Verification items for the finished model (mm, model axes). Coordinates: 2 decimals unless noted, no trailing zeros. Order: outer loops, then holes, each group sorted by start corner. A loop starts at its lowest first (then second) coordinate and runs counter-clockwise, first axis right, second up. Notation, with made-up numbers: M -3.75,82 L 32.25,82 A24 cw 32.25,119 Z; hole C 75,5.5 d4. An arc over 180 degrees is marked long. Return JSON: item names as keys, results as strings.
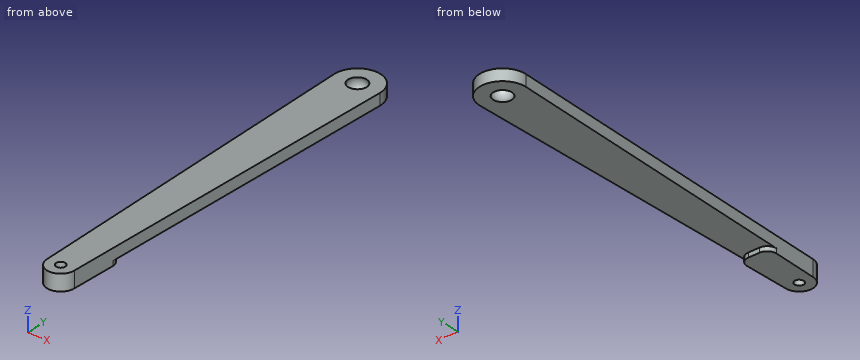
Autodesk Inventor part; units mm, degrees
ref_plane "YZ Plane" through (0, 0, 0) normal (1, 0, 0) x (0, 1, 0)
ref_plane "XZ Plane" through (0, 0, 0) normal (0, 1, 0) x (-1, 0, 0)
ref_plane "XY Plane" through (0, 0, 0) normal (0, 0, 1) x (1, 0, 0)
sketch "Sketch1" plane through (0, 0, 0) normal (0, 0, 1) x (1, 0, 0)
  circle A0 centre (0, 0) radius 0.5
  spline S0 degree 3 poles (0.2195, 78.8895) (0.2199, 78.9523) (0.2329, 79.0192) (0.2847, 79.142) (0.3236, 79.198) (0.413, 79.2862) (0.4694, 79.3243) (0.5929, 79.3745) (0.66, 79.3866) (0.7856, 79.3858) (0.8524, 79.3728) (0.9753, 79.321) (1.0313, 79.2822) (1.1195, 79.1928) (1.1576, 79.1363) (1.2078, 79.0128) (1.2199, 78.9458) (1.2191, 78.8202) (1.2061, 78.7533) (1.1543, 78.6305) (1.1154, 78.5745) (1.0261, 78.4863) (0.9696, 78.4482) (0.8461, 78.398) (0.779, 78.3858) (0.6535, 78.3867) (0.5866, 78.3996) (0.4637, 78.4515) (0.4078, 78.4903) (0.3196, 78.5797) (0.2815, 78.6362) (0.2312, 78.7597) (0.2191, 78.8267) (0.2195, 78.8895) knots 0 0 0 0 0.0625 0.0625 0.125 0.125 0.1875 0.1875 0.25 0.25 0.3125 0.3125 0.375 0.375 0.4375 0.4375 0.5 0.5 0.5625 0.5625 0.625 0.625 0.6875 0.6875 0.75 0.75 0.8125 0.8125 0.875 0.875 0.9375 0.9375 1 1 1 1
  line L0 (0.6862, 78.8895) -> (0, 0)
  circle A1 centre (0, 0) radius 3
  circle A2 centre (0.6862, 78.8895) radius 5
  line L1 (5.6833, 78.7193) -> (2.9983, -0.1021)
  line L2 (-2.9996, -0.05) -> (-4.3131, 78.8063)
  circle A3 centre (0, 0) radius 0.75
  point P0 (0, 0)
  point P1 (0.2195, 78.8895)
  dimension "d0" = 6
  dimension "d1" = 10
  dimension "d12" = 1.5
extrude "Extrusion1" add sketch "Sketch1" along normal blind 3.5 contours A2 L1 A1 L0 | L0 A1 L2 A2 | A2 | A1 | A3
sketch "Sketch2" plane through (5.6833, 78.7193, 3.5) normal (0.9994203, -0.0340447, 0) x (0, 0, -1)
  line L0 (3.5, -66.8672) -> (2.5, -66.8672)
  line L1 (2.5, -66.8672) -> (2.5, 7.5211)
  line L2 (2.5, 7.5211) -> (3.5, 7.5211)
  line L3 (3.5, 7.5211) -> (3.5, -66.8672)
  line L4 (3.5, -81.8672) -> (0, -81.8672)
  line L5 (3.5, -78.8672) -> (3.5, 0)
  dimension "d4" = 1
  dimension "d5" = 15
extrude "Extrusion2" cut sketch "Sketch2" against normal through all
fillet "Fillet1" radius 2 2 edges at (3.4068, 11.8909, 0.5) (-3.2022, 12.116, 0.5)
ref_plane "Work Plane1" through (0.6862, 78.8895, 2.25) normal (0, 0, -1) x (-0.9999622, 0.0086975, 0)
sketch "Sketch3" plane through (0.6862, 78.8895, 2.25) normal (0, 0, -1) x (-0.9999622, 0.0086975, 0)
  arc A0 (0, -2.375) -> (0, 2.375) centre (0, 0) ccw
  line L0 (0, 2.375) -> (0, -2.375)
  point P0 (0, -78.8925)
  dimension "d10" = 4.75
revolve "Revolution1" cut sketch "Sketch3" angle 360 about axis through (0.7068, 81.2645, 2.25) along (-0.0086975, -0.9999622, 0)
sketch "Sketch4" plane through (0, 0, 3.5) normal (0, 0, 1) x (1, 0, 0)
  circle A0 centre (0, 0) radius 0.5
  circle A1 centre (0, 0) radius 1
  point P0 (0, 0)
  dimension "d13" = 2
extrude "Extrusion3" cut sketch "Sketch4" against normal through all
properties part number "RightArm"
Q1. Go/stop test with flat-tipped pins: pin 1 (5 mm diameter, centred on x = 4, y = 45.5, fed in from -Z); pin 2 (3.5 mm diameter, centred on x = 1, y = 1.5, fed in from -Z); pin 3 (5 mm diameter, centred on x = 0, y = 40.5, fed in from +Z). Record where each tip stops, or that it passes through.
Values:
{"pin 1": "z = 1", "pin 2": "z = 0", "pin 3": "z = 3.5"}
Q2. Cross-section at B-B, the plane y = 73. Record the boundary of the cut face in (x, z).
Values:
{"outline": "M -4.22,1 L 5.49,1 L 5.49,3.5 L -4.22,3.5 Z"}
Q3. Material ranges on line 1 along Y through (x, z) = (0, 2.65); line 2 along Y through (x, z) = (0, 2.3); line 3 along Z through (x, y) = (-1, 41), recorded low to high.
Values:
{"line 1": "-3 to -1, 1 to 76.65, 81.13 to 83.84", "line 2": "-3 to -1, 1 to 76.62, 81.16 to 83.84", "line 3": "1 to 3.5"}
Q4. Cross-section at A-A, the plane x = 4.75. Record the boundary of the cut face in (y, z).
Values:
{"outline": "M 51.32,1 L 81.8,1 L 81.8,3.5 L 51.32,3.5 Z"}
